Design review of the part built by this model. Coordinates are the model's own, in mm. A direction names the side the tool comes from. Coordinates: 2 decimals unless noted, no trailing zeros. Order: outer loops, then holes, each group sorted by start corner. A loop starts at its lowest first (then second) coordinate and runs counter-clockwise, first axis right, second up. Notation, with made-up numbers: M 61,44 L 115,44 A30 cw 115,78 Z; hole C 1,52 d6. An arc over 180 degrees is marked long. Use CSV: the item, a comma, the result in double quotes.
```python
from build123d import *

# Parameters (mm, degrees)
SKETCH2_W           = 20
SKETCH2_H           = 20
BOSS_EXTRUDE2_DEPTH = 40
SKETCH4_W           = 5
SKETCH4_H           = 10
CUT_EXTRUDE1_DEPTH  = 41
CIRPATTERN1_COUNT   = 4
SKETCH10_W          = 20
SKETCH10_H          = 15
BOSS_EXTRUDE4_DEPTH = 15
CUT_EXTRUDE3_DEPTH  = 21
SKETCH13_W          = 20
SKETCH13_H          = 25
CUT_EXTRUDE4_DEPTH  = 21


with BuildPart() as part:
    # Sketch2 → Boss-Extrude2 (new body)
    with BuildSketch(Plane(origin=(0, 0, 0), x_dir=(1, 0, 0), z_dir=(0, 1, 0))):
        Rectangle(SKETCH2_W, SKETCH2_H)
    extrude(amount=BOSS_EXTRUDE2_DEPTH)

    # Sketch4 → Cut-Extrude1 (cut, through all)
    with BuildSketch(Plane.XZ):
        with Locations((0, 10)):
            Rectangle(SKETCH4_W, SKETCH4_H)
    cut_extrude1 = extrude(amount=-CUT_EXTRUDE1_DEPTH, mode=Mode.SUBTRACT)

    # CirPattern1: Cut-Extrude1 ×4 about axis
    cirpattern1_axis = Axis((0, 0, -0.5), (0, 1, 0))
    for i in range(1, CIRPATTERN1_COUNT):
        add(cut_extrude1.rotate(cirpattern1_axis, i * 360 / CIRPATTERN1_COUNT), mode=Mode.SUBTRACT)

    # Sketch10 → Boss-Extrude4 (add)
    with BuildSketch(Plane(origin=(0, 0, -10), x_dir=(-1, 0, 0), z_dir=(0, 0, -1))):
        with Locations((0, 32.5)):
            Rectangle(SKETCH10_W, SKETCH10_H)
    extrude(amount=BOSS_EXTRUDE4_DEPTH)

    # Sketch12 → Cut-Extrude3 (cut, through all)
    with BuildSketch(Plane.ZY.offset(10)):
        Polygon((-25, 40), (-10, 25), (-25, 25), align=None)
    extrude(amount=-CUT_EXTRUDE3_DEPTH, mode=Mode.SUBTRACT)

    # Sketch13 → Cut-Extrude4 (cut, through all)
    with BuildSketch(Plane.ZY.offset(10)):
        with Locations((0, 12.5)):
            Rectangle(SKETCH13_W, SKETCH13_H)
    extrude(amount=-CUT_EXTRUDE4_DEPTH, mode=Mode.SUBTRACT)


solid = part.part
```
(1) Wall thickness on probe 1 along X at (y, z) = (37.5, 8); probe 2 along Z at (x, y) = (8, 37.5); probe 3 along Z at (x, y) = (-0.75, 35): over which ranges is each line inside the solid? List them lowest first.
The answers:
probe 1,"x = -10 to -2.5, 2.5 to 10"
probe 2,"z = -22.5 to -3, 2 to 10"
probe 3,"z = -20 to -10, -6 to 5"
(2) Add section C-C on x = 1. State the section outline as (y, z) points, and give its area (4 significant figures).
The answers:
outline,"M 25,-10 L 40,-25 L 40,-10 Z; M 25,-6 L 40,-6 L 40,5 L 25,5 Z"
area,"277.5 mm2"
(3) For faces 4 (the face through (8, 32, -3)), 5 (the face through (-2.5, 32, 7)), 6 (the face through (-2.5, 32, -8)), list the 3-axis set-ups (+Z, -Z, +X, -X, +Y, -Y) from which the entire face can be reached by the end or side of a thin tool; tool diameter is ignored.
The answers:
face 4,"+X, +Y, -Y"
face 5,"+Z, +Y, -Y"
face 6,"+Y, -Y"
(4) Clearance check with flat-ended pins moving along their axes: P1, Ø2, axis at x = 7, y = 33.5, coming from the -Z side; P2, Ø1.5, axis at x = 1, y = 29.5, coming from the -Z side; P3, Ø4, axis at x = -5.5, y = 33.5, coming from the -Z side. State where each tip first meets the part, or that it passes through.
The answers:
P1,"stops at z = -19.5"
P2,"stops at z = -15.25"
P3,"stops at z = -20.5"
(5) Add section B-B on y = 35.75. State the section outline as (x, z) points, and give its area (3 significant figures).
The answers:
outline,"M -10,-20.75 L 10,-20.75 L 10,-3 L 5.5,-3 L 5.5,2 L 10,2 L 10,10 L 2.5,10 L 2.5,5 L -2.5,5 L -2.5,10 L -10,10 L -10,2 L -5.5,2 L -5.5,-3 L -10,-3 Z; hole M -2.5,-10 L 2.5,-10 L 2.5,-6 L -2.5,-6 Z"
area,"525 mm2"
(6) Add section D-D on y = 28.25. State the section outline as (x, z) points, and give its area (3 significant figures).
The answers:
outline,"M -10,-13.25 L 10,-13.25 L 10,-3 L 5.5,-3 L 5.5,2 L 10,2 L 10,10 L 2.5,10 L 2.5,5 L -2.5,5 L -2.5,10 L -10,10 L -10,2 L -5.5,2 L -5.5,-3 L -10,-3 Z; hole M -2.5,-10 L 2.5,-10 L 2.5,-6 L -2.5,-6 Z"
area,"375 mm2"
(7) The part is to be moulded in two halves that separate along X. For faces 1 (the face through (-6, 32, 10)), 2 (the face through (2.5, 32, -8)), 3 (the face through (-10, 32, 6)), say which applies: pulls with the +X half, pulls with the -X half, needs draft (parallel to the pull), parting line crosses it, or undercut.
The answers:
face 1,"needs draft"
face 2,"undercut"
face 3,"pulls with the -X half"
(8) Add section A-A on z = -6.5. State the section outline as (x, y) points, and give its area (3 significant figures).
The answers:
outline,"M -10,25 L -2.5,25 L -2.5,40 L -10,40 Z; M 2.5,25 L 10,25 L 10,40 L 2.5,40 Z"
area,"225 mm2"
